Autodesk Inventor part; units mm, degrees
ref_plane "YZ Plane" through (0, 0, 0) normal (1, 0, 0) x (0, 1, 0)
ref_plane "XZ Plane" through (0, 0, 0) normal (0, 1, 0) x (-1, 0, 0)
ref_plane "XY Plane" through (0, 0, 0) normal (0, 0, 1) x (1, 0, 0)
sketch "スケッチ1" plane through (0, 0, 0) normal (0, 0, 1) x (1, 0, 0)
  line L0 (-12.5, 36) -> (12.5, 36)
  line L1 (12.5, 36) -> (12.5, -48)
  line L2 (12.5, -48) -> (-12.5, -48)
  line L3 (-12.5, -48) -> (-12.5, 36)
  point P0 (0, 0)
  dimension "d0" = 36
  dimension "d1" = 25
  dimension "d2" = 12.5
  dimension "d3" = 48
extrude "押し出し1" add sketch "スケッチ1" along normal blind 15
sketch "スケッチ2" plane through (0, 0, 0) normal (0, 0, -1) x (-1, 0, 0)
  line L0 (-12.5, 36) -> (-12.5, -48)
  line L1 (12.5, -48) -> (12.5, 36)
  line L2 (-12.5, 36) -> (12.5, 36)
  line L3 (12.5, 36) -> (12.5, 24)
  line L4 (12.5, 24) -> (-12.5, 24)
  line L5 (-12.5, 24) -> (-12.5, 36)
  line L6 (12.5, 0) -> (-12.5, 0)
  line L7 (-12.5, 0) -> (-12.5, 12)
  line L8 (-12.5, 12) -> (12.5, 12)
  line L9 (12.5, 12) -> (12.5, 0)
  point P0 (0, 0)
  dimension "d6" = 12
  dimension "d42" = 12
  dimension "d66" = 12
extrude "押し出し2" cut sketch "スケッチ2" against normal blind 2 contours L2 L1 L4 L0 | L8 L1 L6 L0
sketch "スケッチ3" plane through (0, 0, 2) normal (0, 0, -1) x (-1, 0, 0)
  line L0 (12.5, 36) -> (12.5, 24)
  line L1 (-12.5, 36) -> (12.5, 36)
  line L2 (-12.5, 24) -> (-12.5, 36)
  point P0 (0, 0)
  point P1 (-6.5, 30)
  point P2 (6.5, 30)
  point P3 (12.5, 0)
  point P4 (-12.5, 0)
  dimension "d10" = 6
  dimension "d11" = 6
  dimension "d12" = 6
  dimension "d13" = 6
hole "Hole1" at (6.5, 30, 2) at (-6.5, 30, 2) direction (0, 0, 1) diameter 3.242 end through all
sketch "スケッチ6" plane through (0, 0, 2) normal (0, 0, -1) x (-1, 0, 0)
  line L0 (-12.5, 0) -> (12.5, 0)
  line L1 (12.5, 12) -> (12.5, 0)
  line L2 (-12.5, 0) -> (-12.5, 12)
  point P0 (0, 0)
  point P1 (-6.5, 6)
  point P2 (6.5, 6)
  dimension "d43" = 6
  dimension "d44" = 6
  dimension "d45" = 6
  dimension "d46" = 6
hole "Hole4" at (6.5, 6, 2) at (-6.5, 6, 2) direction (0, 0, 1) diameter 3.242 end through all
sketch "スケッチ7" plane through (0, 0, 0) normal (0, 0, -1) x (-1, 0, 0)
  line L0 (12.5, 24) -> (-12.5, 24)
  line L1 (12.5, 12) -> (12.5, 24)
  point P0 (0, 0)
  point P1 (0, 18)
  dimension "d54" = 6
  dimension "d55" = 12.5
hole "Hole5" at (0, 18, 0) direction (0, 0, 1) diameter 8 end through all
sketch "スケッチ8" plane through (0, 0, 0) normal (0, 0, -1) x (-1, 0, 0)
  line L0 (12.5, 0) -> (-12.5, 0)
  line L1 (-12.5, 0) -> (-12.5, -48)
  line L2 (-12.5, -48) -> (12.5, -48)
  line L3 (12.5, -48) -> (12.5, 0)
  line L4 (0, 0) -> (0, -48)
  line L5 (12.5, -24) -> (-12.5, -24)
  line L6 (-9.85, -3.15) -> (9.85, -3.15)
  line L7 (9.85, -3.15) -> (9.85, -39.05)
  line L8 (9.85, -39.05) -> (-9.85, -39.05)
  line L9 (-9.85, -39.05) -> (-9.85, -3.15)
  dimension "d63" = 19.7
  dimension "d64" = 19.7
  dimension "d65" = 35.9
  dimension "d68" = 3.15
extrude "押し出し3" cut sketch "スケッチ8" against normal through all contours L6 L7 L5 L4 | L4 L5 L9 L6 | L7 L8 L4 L5 | L4 L8 L9 L5
fillet "フィレット2" radius 5.05 2 edges at (9.85, -3.15, 7.5) (-9.85, -3.15, 7.5)
fillet "フィレット3" radius 3.05 2 edges at (9.85, -39.05, 7.5) (-9.85, -39.05, 7.5)
fillet "フィレット4" radius 12.5 2 edges at (12.5, -48, 7.5) (-12.5, -48, 7.5)
sketch "スケッチ13" plane through (0, 0, 15) normal (0, 0, 1) x (1, 0, 0)
  arc A0 (-12.5, -35.5) -> (12.5, -35.5) centre (0, -35.5) ccw
  line L0 (12.5, 36) -> (12.5, -35.5)
  line L1 (-12.5, 36) -> (12.5, 36)
  line L2 (-12.5, -35.5) -> (-12.5, 36)
  circle A1 centre (-6.5, 6) radius 1.621
  circle A2 centre (6.5, 6) radius 1.621
  point P0 (0, 0)
  point P1 (-10, 33.5)
  point P2 (10, 33.5)
  point P3 (-10, 3)
  point P4 (10, 3)
  point P5 (-5, -43)
  point P6 (5, -43)
  dimension "d106" = 2.5
  dimension "d107" = 2.5
  dimension "d108" = 2.5
  dimension "d109" = 2.5
  dimension "d110" = 2.5
  dimension "d111" = 2.5
  dimension "d112" = 3
  dimension "d113" = 3
  dimension "d114" = 5
  dimension "d115" = 5
  dimension "d125" = 79
  dimension "d126" = 79
hole "Hole8" at (-10, 33.5, 15) at (10, 33.5, 15) at (-10, 3, 15) at (10, 3, 15) at (-5, -43, 15) at (5, -43, 15) direction (0, 0, -1) diameter 1.567 end through all
sketch "スケッチ14" plane through (0, 0, 0) normal (0, 0, -1) x (-1, 0, 0)
  circle A0 centre (0, 18) radius 4
  line L0 (12.5, 24) -> (-12.5, 24)
  line L1 (-12.5, 24) -> (-12.5, 12)
  line L2 (-12.5, 12) -> (12.5, 12)
  line L3 (12.5, 12) -> (12.5, 24)
  line L4 (-10.4, 24) -> (10.4, 24)
  line L5 (10.4, 24) -> (10.4, 12)
  line L6 (10.4, 12) -> (-10.4, 12)
  line L7 (-10.4, 12) -> (-10.4, 24)
  point P0 (0, 0)
  dimension "d127" = 2.1
  dimension "d128" = 2.1
extrude "押し出し4" add sketch "スケッチ14" along normal blind 5 contours L5 L2 L7 L0
equation "\"d42\" = d6"
equation "\"d66\" = d42"
equation "\"d64\" = d63"
equation "\"d128\" = d127"
properties part number "JointC3'_2nd" material "ポリプロピレン"
The listing builds one solid part. Answer for the finished solid, in the listing's coordinates (mm). A direction names the side the tool comes from. Round coordinates to 2 decimals unless told otherwise and drop trailing zeros. Loops run counter-clockwise (first coordinate to the right, second up) from the corner with the lowest first, then second, coordinate; pieces in that order, holes last.
1) A cutting plane is placed at A-A on y = 6. Determine the outline of the cut face in (x, z), plus the area to 3 significant figures.
Outcome:
outline: (-12.5, 2) - (-8.12, 2) - (-8.12, 15) - (-12.5, 15) - close; (-4.88, 2) - (4.88, 2) - (4.88, 15) - (-4.88, 15) - close; (8.12, 2) - (12.5, 2) - (12.5, 15) - (8.12, 15) - close
area: 241 mm2
2) A cutting plane is placed at D-D on x = 3.25. Determine the outline of the cut face in (y, z), plus the area to 3 significant figures.
Outcome:
outline: (-47.57, 0) - (-39.05, 0) - (-39.05, 15) - (-47.57, 15) - close; (-3.15, 0) - (0, 0) - (0, 2) - (12, 2) - (12, -5) - (15.67, -5) - (15.67, 15) - (-3.15, 15) - close; (20.33, -5) - (24, -5) - (24, 2) - (36, 2) - (36, 15) - (20.33, 15) - close
area: 634 mm2
3) Given P1, Ø5, axis at x = -6.5, y = 6, coming from the -Z side; P2, Ø3, axis at x = 4, z = 3.5, coming from the -Y side; P3, Ø1, axis at x = -8.5, z = 9.5, coming from the -Y side, each flat-ended and moving along its own axis, determine where each tip first touches the part or whether it passes through.
Outcome:
P1: stops at z = 2
P2: stops at y = -47.75
P3: stops at y = -45.1
4) A cutting plane is placed at C-C on y = -10.5. Determine the outline of the cut face in (x, z), plus the area to 3 significant figures.
Outcome:
outline: (-12.5, 0) - (-9.85, 0) - (-9.85, 15) - (-12.5, 15) - close; (9.85, 0) - (12.5, 0) - (12.5, 15) - (9.85, 15) - close
area: 79.5 mm2
5) Consider line 1 (X direction, y = 3, z = 8.75); line 2 (X direction, y = 6, z = 10); line 3 (Y direction, x = 10, z = 9.5). Determine where each line is inside the solid, lowest interval first.
Outcome:
line 1: x = -12.5 to -10.78, -9.22 to 9.22, 10.78 to 12.5
line 2: x = -12.5 to -8.12, -4.88 to 4.88, 8.12 to 12.5
line 3: y = -43 to 2.22, 3.78 to 32.72, 34.28 to 36
6) For faces 4 (the face through (-10.4, 18, -2)), 5 (the face through (-8.33, -4.59, 7.6)), 6 (the face through (0, 24, -1)), 7 (the face through (0, 12, -1)), determine the directions among +Z, -Z, +X, -X, +Y, -Y from which every point of the face is accessible in a straight line to the end or side of a thin tool.
Outcome:
face 4: -Z, -X, +Y, -Y
face 5: +Z, -Z
face 6: -Z, +X, -X, +Y
face 7: -Z, +X, -X
7) For a pull along Y with two mould halves and no side action, classify faces 1 (the face through (8.741, -44.436, 7.605)), 2 (the face through (10.765, 3.17, 8.409)), 3 (the face through (11, 18, 0)) as released by +Y, released by -Y, zero draft, split by the parting line, or undercut.
Outcome:
face 1: released by -Y
face 2: undercut
face 3: zero draft
8) A cutting plane is placed at B-B on z = -3. Determine the outline of the cut face in (x, y).
Outcome:
outline: (-10.4, 12) - (10.4, 12) - (10.4, 24) - (-10.4, 24) - close; hole circle Ø8 at (0, 18)
